Work out the finished part from the listing and answer in its coordinate system (mm). Face numbers are marked on the shaded views. A direction names the side the tool comes from. Coordinates: 2 decimals unless noted, no trailing zeros. Loops run counter-clockwise (first coordinate to the right, second up) from the corner with the lowest first, then second, coordinate; pieces in that order, holes last. Notation, with made-up numbers: M -0.5,-25 L 19.5,-25 A19 ccw 19.5,11 Z; hole C 17.5,42 d2. An arc over 180 degrees is marked long. Write each question's results on one line, items separated by ' | '.
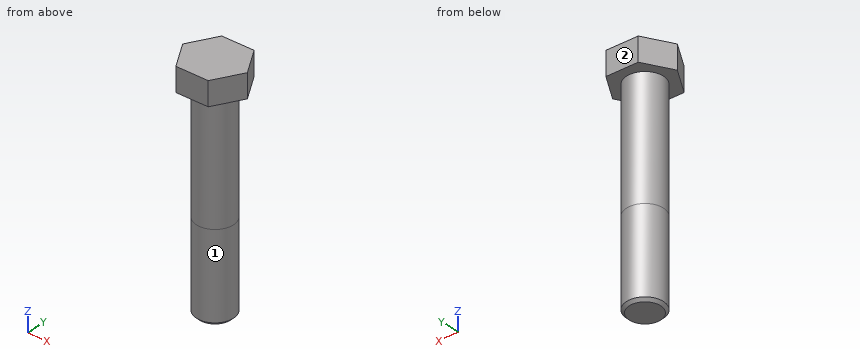
Solid Edge part; units mm, degrees
sketch "Sketch1" plane through (0, 0, 0) normal (0, 0, 1) x (1, 0, 0)
  circle A0 centre (0, 0) radius 13.92
extrude "Protrusion1" add sketch "Sketch1" along normal blind 10.32
sketch "Sketch2" plane through (0, 0, 0) normal (0, 0, -1) x (1, 0, 0)
  circle A0 centre (0, 0) radius 8
extrude "Protrusion2" add sketch "Sketch2" along normal blind 90
sketch "Sketch3" plane through (0, 0, -90) normal (0, 0, -1) x (1, 0, 0)
  circle A0 centre (0, 0) radius 7.9997
extrude "Cutout1" cut sketch "Sketch3" against normal blind 38 flip side to cut
chamfer "Chamfer_1" distance 1.2 angle 45 1 edges at (-7.9997, 0, -90)
sketch "Sketch4" plane through (0, 0, 10.32) normal (0, 0, 1) x (1, 0, 0)
  line L0 (-7.0545, 12) -> (7.0545, 12)
extrude "Cutout2" cut sketch "Sketch4" against normal up to next material side at (0, 12.05, 10.32)
pattern_circular "Pattern1" count 6 over 360 about axis through (0, 0, 10.32) along (0, 0, 1) of "Cutout2"
properties part number "118589" material "Stainless Steel, 304"
1) Which of the six approach directions +Z, -Z, +X, -X, +Y, -Y give full straight-line access (tool end or side, diameter ignored) to the marked faces 1 and 2?
Check result:
face 1: -Z | face 2: +Z, -Z, +X, -X, +Y
2) Straight lines are drawn through the part: probe 1 along Z at (x, y) = (6.5, -7.5); probe 2 along Y at (x, z) = (0.5, -82). For each, find the intervals that lie inside material, in ascending order. Write a range as [from, to].
Check result:
probe 1: [0, 10.32] | probe 2: [-7.98, 7.98]
3) Given pin 1 Ø3 at (x, z) = (7, -25.5) entering from +Y; pin 2 Ø4 at (x, z) = (-6.5, -66) entering from -Y; pin 3 Ø12 at (x, z) = (-7, -72.5) entering from -Y, each flat-ended and moving along its own axis, determine where each tip first touches the part or whether it passes through.
Check result:
pin 1: y = 5.81 | pin 2: y = -6.61 | pin 3: y = -7.94
4) Find section C-C, the plane y = 10. Give the vertices of the cut face in (x, z).
Check result:
outline: M -8.08,0 L 8.08,0 L 8.08,10.32 L -8.08,10.32 Z
5) Find section B-B, the plane z = -45.5. Give the vertices of the cut face in (x, y), and give its area (3 significant figures).
Check result:
outline: C 0,0 d16 | area: 201 mm^2
